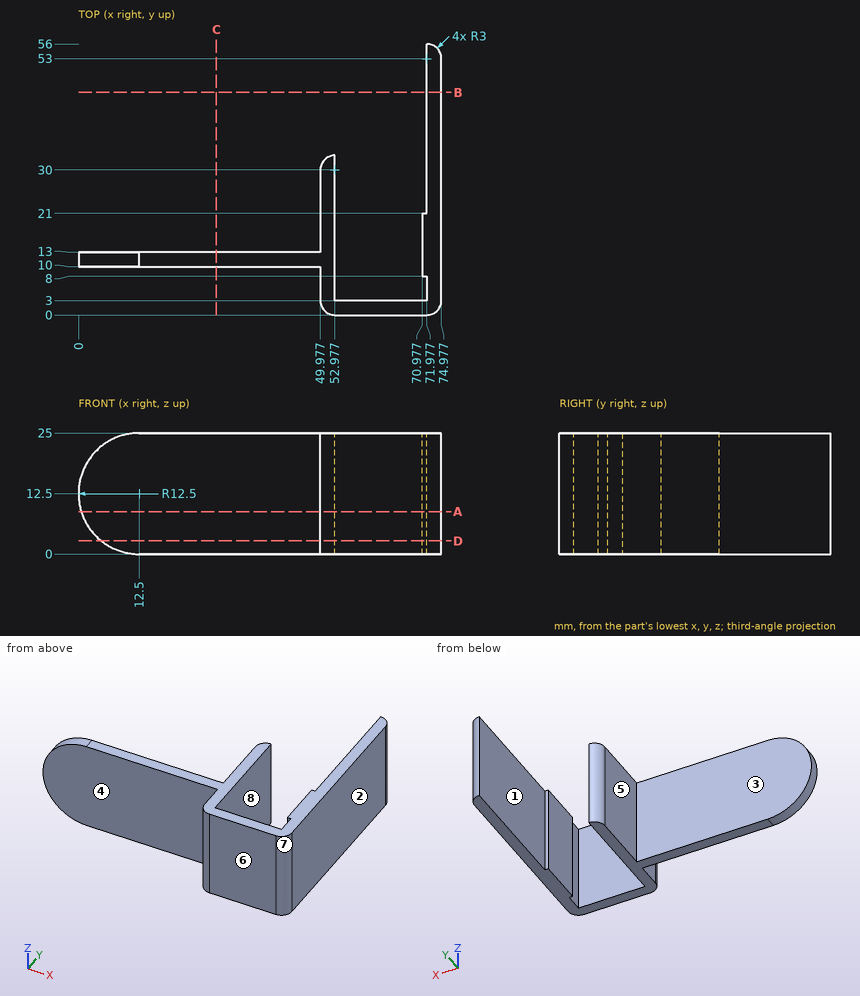
Geometry check sheet. Reference: drawing and pictorial views, mm from the part's lowest x, y, z. A direction names the side the tool comes from. Give positions to 0.01 mm unless a question says otherwise; leave off trailing zeros. Loops run counter-clockwise (first coordinate to the right, second up) from the corner with the lowest first, then second, coordinate; pieces in that order, holes last. Notation, with made-up numbers: M -9,38 L 4,38 A32 ccw 4,69 Z; hole C 54.25,5.5 d3. An arc over 180 degrees is marked long. Use a Markdown table: item, result. Add a question column.
Q1. Sectioned sample at D-D, the plane z = 2.75. Record the cut outline in (x, y), then the cut area to 3 significant figures.
Q2. Sectioned sample at A-A, the plane z = 8.75. Record the cut outline in (x, y).
Q3. Go/stop test with flat-tipped pins: pin 1 (15 mm diameter, centred on x = 62, z = 12, fed in from +Y); pin 2 (4 mm diameter, centred on y = 6, z = 11, fed in from -X); pin 3 (5 mm diameter, centred on x = 67, y = 43, fed in from -Z); pin 4 (6 mm diameter, centred on x = 50, z = 3, fed in from +Y). Record where each tip stops, or that it passes through.
Q4. Sectioned sample at B-B, the plane y = 46. Record the cut outline in (x, z), then the cut area to 3 significant figures.
Q5. Mould release check, pull along X, two halves, no side actions. Record for the marked faces 5, 6, 7 and 8: pulls with the +X half, pulls with the -X half, needs draft (parallel to the pull), parting line crosses it, or undercut.
Q6. Scan lines: line 1 along X through (y, z) = (14, 7.25); line 2 along X through (y, z) = (45, 19.5); line 3 along Y through (x, z) = (68, 3.25). Record each from-to range of solid material in increasing order. Write a range as [from, to].
Q7. Sectioned sample at C-C, the plane x = 28.5. Record the cut outline in (y, z), then the cut area to 3 significant figures.
Q8. Tool access check on the marked faces 1, 2, 3 and 4. Record the directions out of +Z, -Z, +X, -X, +Y, -Y that give a thin tool (end or side, any length) a straight path to the whole face; none if there is none.
Verdict:
| question | item | result |
|---|---|---|
| 1 | outline | M 4.68,10 L 49.98,10 L 49.98,3 A3 ccw 52.98,0 L 71.98,0 A3 ccw 74.98,3 L 74.98,53 A3 ccw 71.98,56 L 71.98,21 L 70.98,21 L 70.98,8 L 71.98,8 L 71.98,3 L 52.98,3 L 52.98,33 A3 ccw 49.98,30 L 49.98,13 L 4.68,13 Z |
| 1 | area | 465 mm^2 |
| 2 | outline | M 0.58,10 L 49.98,10 L 49.98,3 A3 ccw 52.98,0 L 71.98,0 A3 ccw 74.98,3 L 74.98,53 A3 ccw 71.98,56 L 71.98,21 L 70.98,21 L 70.98,8 L 71.98,8 L 71.98,3 L 52.98,3 L 52.98,33 A3 ccw 49.98,30 L 49.98,13 L 0.58,13 Z |
| 3 | pin 1 | y = 3 |
| 3 | pin 2 | x = 49.98 |
| 3 | pin 3 | through |
| 3 | pin 4 | y = 33 |
| 4 | outline | M 71.98,0 L 74.98,0 L 74.98,25 L 71.98,25 Z |
| 4 | area | 75.0 mm^2 |
| 5 | face 5 | pulls with the -X half |
| 5 | face 6 | needs draft |
| 5 | face 7 | pulls with the +X half |
| 5 | face 8 | undercut |
| 6 | line 1 | [49.98, 52.98], [70.98, 74.98] |
| 6 | line 2 | [71.98, 74.98] |
| 6 | line 3 | [0, 3] |
| 7 | outline | M 10,0 L 13,0 L 13,25 L 10,25 Z |
| 7 | area | 75.0 mm^2 |
| 8 | face 1 | +Z, -Z, +Y |
| 8 | face 2 | +Z, -Z, +X, +Y, -Y |
| 8 | face 3 | +Z, -Z, -X, +Y |
| 8 | face 4 | +Z, -Z, -X, -Y |
